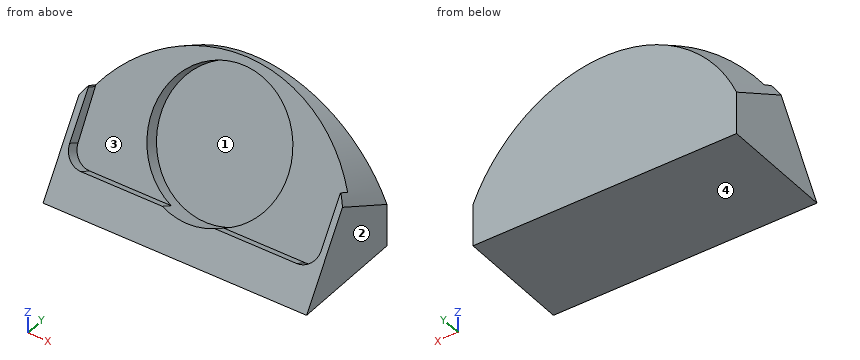
```python
from build123d import *

# Parameters (mm, degrees)
PAD_DEPTH       = 88
POCKET_DEPTH    = 11
SKETCH011_R     = 46
POCKET001_DEPTH = 10.5
POCKET002_DEPTH = 66.2698164218
POCKET003_DEPTH = 10


with BuildPart() as part:
    # Sketch → Pad (new body, symmetric)
    with BuildSketch(Plane.YZ):
        Polygon((0, 0), (65.2925492254, 100.9999079658), (76.520638, 100.9999079658), (76.520638, 0), align=None)
    extrude(amount=PAD_DEPTH, both=True)

    # Sketch010 (on DatumPlane) → Pocket (cut)
    with BuildSketch(Plane(origin=(0, 54.6423048454, 94.6432482349), x_dir=(1, 0, 0), z_dir=(0, -0.8660254038, 0.5))):
        with BuildLine():
            Line((-84, 85), (-84, -73))
            ThreePointArc((-84, -73), (-80.4852813742, -81.4852813742), (-72, -85))
            Line((-72, -85), (72, -85))
            ThreePointArc((72, -85), (80.4852813742, -81.4852813742), (84, -73))
            Line((84, -73), (84, 85))
            Line((84, 85), (-84, 85))
        make_face()
    extrude(amount=-POCKET_DEPTH, mode=Mode.SUBTRACT)

    # Sketch011 (on Face12 of Pocket) → Pocket001 (cut, symmetric)
    with BuildSketch(Plane(origin=(0, 9.5262794416, -5.5), x_dir=(1, 0, 0), z_dir=(0, -0.8660254038, 0.5))):
        with Locations((0, 66.7846096908)):
            Circle(SKETCH011_R)
    extrude(amount=POCKET001_DEPTH, both=True, mode=Mode.SUBTRACT)

    # Sketch012 (on Face14 of Pocket001) → Pocket002 (cut, through all)
    with BuildSketch(Plane(origin=(0, 0, 0), x_dir=(1, 0, 0), z_dir=(0, -0.8660254038, 0.5))):
        with BuildLine():
            ThreePointArc((97.8966291555, 24.2846096908), (0, 117.7846096908), (-97.8966291555, 24.2846096908))
            Line((-97.8966291555, 154.2846096908), (-97.8966291555, 24.2846096908))
            Line((97.8966291555, 154.2846096908), (-97.8966291555, 154.2846096908))
            Line((97.8966291555, 24.2846096908), (97.8966291555, 154.2846096908))
        make_face()
    extrude(amount=-POCKET002_DEPTH, mode=Mode.SUBTRACT)

    # Sketch016 (on Face14 of Pocket002) → Pocket003 (cut)
    with BuildSketch(Plane(origin=(0, 9.5262794416, -5.5), x_dir=(1, 0, 0), z_dir=(0, -0.8660254038, 0.5))):
        with BuildLine():
            ThreePointArc((88, 69.0708248262), (86, 71.0708248262), (84, 69.0708248262))
            Line((84, 84.0708248262), (84, 69.0708248262))
            Line((88, 84.0708248262), (84, 84.0708248262))
            Line((88, 69.0708248262), (88, 84.0708248262))
        make_face()
        with BuildLine():
            ThreePointArc((-84, 69.0708248262), (-86, 71.0708248262), (-88, 69.0708248262))
            Line((-88, 85.0708248262), (-88, 69.0708248262))
            Line((-84, 85.0708248262), (-88, 85.0708248262))
            Line((-84, 69.0708248262), (-84, 85.0708248262))
        make_face()
    extrude(amount=POCKET003_DEPTH, mode=Mode.SUBTRACT)


solid = part.part
```
Part model, mm, in its own coordinate system. Face numbers are marked on the shaded views. Coordinates: 2 decimals unless noted, no trailing zeros. Order: outer loops, then holes, each group sorted by start corner. A loop starts at its lowest first (then second) coordinate and runs counter-clockwise, first axis right, second up. Notation, with made-up numbers: (-25, 18.5) -> (21, 18.5) arc R9 cw to (21, 30.5) -> close; hole circle Ø8 at (-3.75, 86). An arc over 180 degrees is marked (long way). Put each result on its own line as item: value. Start each with the question number.
(1) Band-saw the part on C-C (x = -77). Give the cut face in (y, z).
(2) Probe line 1 along Y through (x, z) = (-8, 14); line 2 along X through (y, z) = (60, 63); line 3 along X through (y, z) = (29, 25). List the from-to ranges inside material, lowest first. Write a range as [from, to].
(3) Pin check, flat tips, straight feed: pin 1 Ø10 at (x, z) = (67, 75.5) entering from +Y; pin 2 Ø10 at (x, y) = (-69, 65.5) entering from +Z. Stop position of each tip, or through.
(4) Band-saw the part on D-D (x = 63). Give the cut face in (y, z), then the cut area to 3 significant figures.
(5) Mould opens along Z. For the marked faces 1, 2, 3 and 4 say: pulls with the +Z half, pulls with the -Z half, needs draft (parallel to the pull), parting line crosses it, or undercut.
(6) Band-saw the part on B-B (x = -35.5). Give the cut face in (y, z).
(7) Band-saw the part on A-A (x = 10). Give the cut face in (y, z).
Determined:
1. outline: (0, 0) -> (76.52, 0) -> (76.52, 48.67) -> (49.73, 64.13) -> (22.21, 16.48) -> (13.79, 21.34) -> close
2. line 1: y = [9.05, 18.72], [32.91, 76.52]
2. line 2: x = [-73.54, -42.43], [42.43, 73.54]
2. line 3: x = [-88, -34.32], [34.32, 88]
3. pin 1: stops at y = 64.27
3. pin 2: stops at z = 71.5
4. outline: (0, 0) -> (76.52, 0) -> (76.52, 65.35) -> (56.95, 76.64) -> (21.67, 15.53) -> (13.2, 20.42) -> close
4. area: 3,300 mm²
5. face 1: undercut
5. face 2: needs draft
5. face 3: pulls with the +Z half
5. face 4: pulls with the -Z half
6. outline: (0, 0) -> (76.52, 0) -> (76.52, 84.14) -> (65.09, 90.74) -> (57.55, 77.67) -> (66.64, 72.42) -> (37.39, 21.75) -> (28.29, 27) -> (21.67, 15.53) -> (13.2, 20.42) -> close
7. outline: (0, 0) -> (76.52, 0) -> (76.52, 91.24) -> (68.16, 96.06) -> (65.37, 91.22) -> (74.46, 85.97) -> (29.56, 8.2) -> (11.9, 18.4) -> close
